from build123d import *

# Parameters (mm, degrees)
SKETCH1_R           = 12.5
BOSS_EXTRUDE1_DEPTH = 32
CHAMFER1_SIZE       = 1


with BuildPart() as part:
    # Sketch1 → Boss-Extrude1 (new body, symmetric)
    with BuildSketch(Plane.XY):
        Circle(SKETCH1_R)
    extrude(amount=BOSS_EXTRUDE1_DEPTH, both=True)

    # Chamfer1
    chamfer1_edges = [part.edges().sort_by_distance(p)[0] for p in [
        (-12.5, 0, -32),
        (-12.5, 0, 32),
    ]]
    chamfer(chamfer1_edges, length=CHAMFER1_SIZE)

    # Sketch4 → Tap Drill for M6 Tap1 (revolve, cut)
    with BuildSketch(Plane(origin=(0, 0, 32), x_dir=(0, -1, 0), z_dir=(1, 0, 0))):
        Polygon((0, 0), (0, 14.502151548), (2.5, 13), (2.5, 0), align=None)
    tap_drill_for_m6_tap1 = revolve(axis=Axis((0, 0, 38.35), (0, 0, -1)), mode=Mode.SUBTRACT)

    # Mirror1: Tap Drill for M6 Tap1 across plane
    add(tap_drill_for_m6_tap1.mirror(Plane.XY), mode=Mode.SUBTRACT)


solid = part.part
Source: CAD feature listing. Evaluate the final solid. Frame: model axes, mm. A direction names the side the tool comes from. Coordinates: 2 decimals unless noted, no trailing zeros. Write each loop counter-clockwise with the first axis right and the second up, starting at its lowest first coordinate (ties: lowest second). Pieces come first, ordered by that corner, then holes. Notation, with made-up numbers: M 2,-16.5 L 35,-16.5 A24 ccw 35,11.5 Z; hole C 69.25,58.25 d8. An arc over 180 degrees is marked long. Use a Markdown table: item, result.
1) Mould query, pull axis X, two halves, no side actions, for faces 3 (the cylindrical face through (2.44, 0.54, 25.59)), 4 (the flat face through (-3, 0, -32)), 5 (the cylindrical face through (11.923, 3.755, 0.434)). Classes: pulls with the +X half, pulls with the -X half, needs draft (parallel to the pull), parting line crosses it, or undercut.
Conclusion:
| item | result |
|---|---|
| face 3 | undercut |
| face 4 | needs draft |
| face 5 | parting line crosses it |
2) Section A-A, the plane z = -7. Output: boundary loops of the cut face in (x, y).
Conclusion:
| item | result |
|---|---|
| outline | C 0,0 d25 |
3) Reachability of faces 1 (the flat face through (-3, 0, 32)), 2 (the cylindrical face through (2.44, 0.54, -25.59)) from +Z, -Z, +X, -X, +Y, -Y: full face, straight path, thin tool, end or side. Return the list, or none.
Conclusion:
| item | result |
|---|---|
| face 1 | +Z, +X, -X, +Y, -Y |
| face 2 | -Z |
4) Ray query, L1, parallel to Y at x = 0, z = 25.5; L2, parallel to Y at x = 0.5, z = -13.5; L3, parallel to X at y = -2.25, z = -14. Return the intervals inside material, ascending.
Conclusion:
| item | result |
|---|---|
| L1 | y = -12.5 to -2.5, 2.5 to 12.5 |
| L2 | y = -12.49 to 12.49 |
| L3 | x = -12.3 to 12.3 |
5) First-contact query: pin 1 Ø2 at (y, z) = (8.5, 5) entering from +X; pin 2 Ø4 at (y, z) = (7, -18) entering from -X; pin 3 Ø6 at (x, z) = (-8, 23) entering from -Y. Flat tips, straight axial feed; report the tip coordinate or a pass-through.
Conclusion:
| item | result |
|---|---|
| pin 1 | stops at x = 10 |
| pin 2 | stops at x = -11.46 |
| pin 3 | stops at y = -11.46 |
